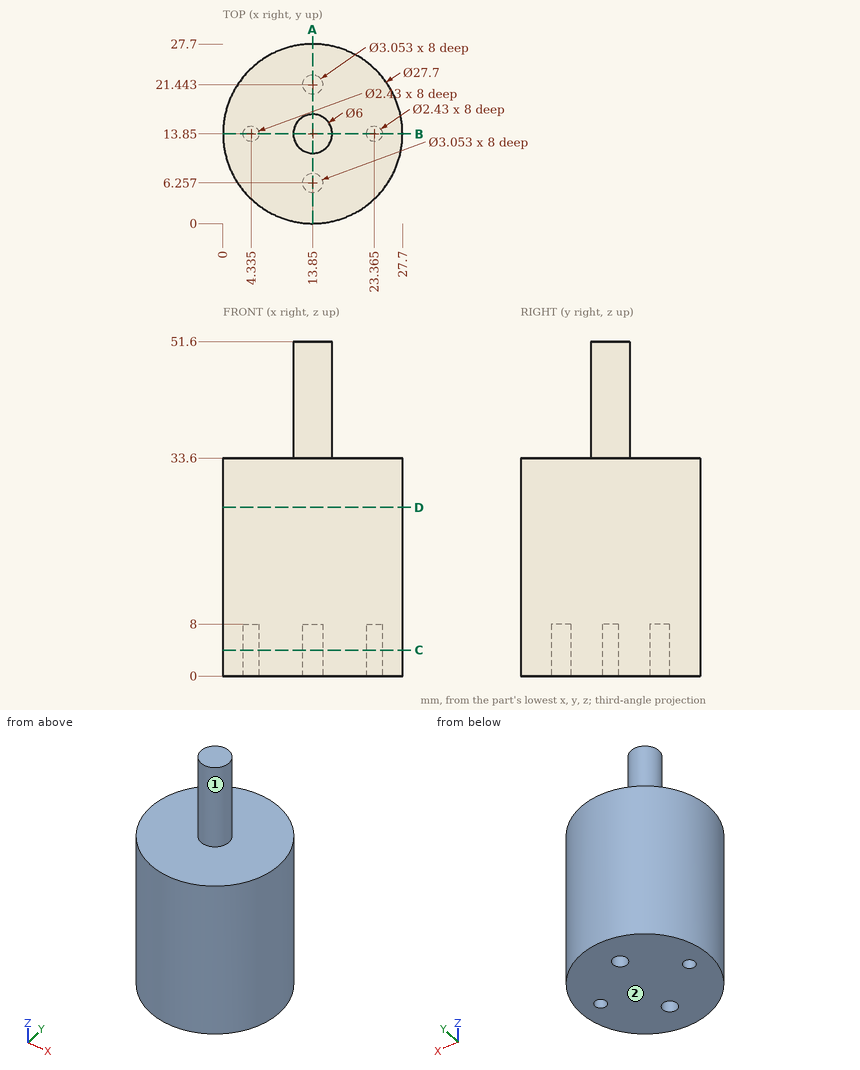
Geometry check sheet. Reference: drawing and pictorial views, mm from the part's lowest x, y, z. A direction names the side the tool comes from. Round coordinates to 2 decimals unless told otherwise and drop trailing zeros. Loops run counter-clockwise (first coordinate to the right, second up) from the corner with the lowest first, then second, coordinate; pieces in that order, holes last. Notation, with made-up numbers: (42, 84.25) -> (72, 84.25) arc R17 ccw to (72, 114.25) -> close; hole circle Ø3 at (-37.75, 5). An arc over 180 degrees is marked (long way). Use a Markdown table: item, result.
(1) Go/stop test with flat-tipped pins: P1, Ø1.5, axis at x = 4.335, y = 13.85, coming from the +Z side; P2, Ø1.2, axis at x = 4.5, y = 14, coming from the -Z side; P3, Ø8, axis at y = 19, z = 42.5, coming from the -X side. Record where each tip stops, or that it passes through.
Calculated:
| item | result |
|---|---|
| P1 | z = 33.6 |
| P2 | z = 8 |
| P3 | x = 11.08 |
(2) Sectioned sample at A-A (x = 13.85). Enter the section's corners in (y, z), then the cut area to 3 significant figures.
Calculated:
| item | result |
|---|---|
| outline | (0, 0) -> (4.73, 0) -> (4.73, 8) -> (7.78, 8) -> (7.78, 0) -> (19.92, 0) -> (19.92, 8) -> (22.97, 8) -> (22.97, 0) -> (27.7, 0) -> (27.7, 33.6) -> (16.85, 33.6) -> (16.85, 51.6) -> (10.85, 51.6) -> (10.85, 33.6) -> (0, 33.6) -> close |
| area | 990 mm² |
(3) Sectioned sample at B-B (y = 13.85). Enter the section's corners in (x, z).
Calculated:
| item | result |
|---|---|
| outline | (0, 0) -> (3.12, 0) -> (3.12, 8) -> (5.55, 8) -> (5.55, 0) -> (22.15, 0) -> (22.15, 8) -> (24.58, 8) -> (24.58, 0) -> (27.7, 0) -> (27.7, 33.6) -> (16.85, 33.6) -> (16.85, 51.6) -> (10.85, 51.6) -> (10.85, 33.6) -> (0, 33.6) -> close |
(4) Set-up check for the marked faces 1 and 2: record each of +Z, -Z, +X, -X, +Y, -Y from which the full face is reachable in a straight line by a thin tool's end or side.
Calculated:
| item | result |
|---|---|
| face 1 | +Z |
| face 2 | -Z, +X, -X, +Y, -Y |
(5) Sectioned sample at D-D (z = 26). Enter the section's corners in (x, y).
Calculated:
| item | result |
|---|---|
| outline | circle Ø27.7 at (13.85, 13.85) |
(6) Scan lines: probe 1 along Y at (x, z) = (13.85, 5.5); probe 2 along Z at (x, y) = (20.75, 8.25); probe 3 along Y at (x, z) = (22.25, 20.5). Record each from-to range of solid material in increasing order.
Calculated:
| item | result |
|---|---|
| probe 1 | 0 to 4.73, 7.78 to 19.92, 22.97 to 27.7 |
| probe 2 | 0 to 33.6 |
| probe 3 | 2.84 to 24.86 |
(7) Sectioned sample at C-C (z = 4). Give the number of separate pieces and of enclosed holes in the cut face, then the cut area to 3 significant figures.
Calculated:
| item | result |
|---|---|
| separate pieces | 1 |
| enclosed holes | 4 |
| area | 579 mm² |
